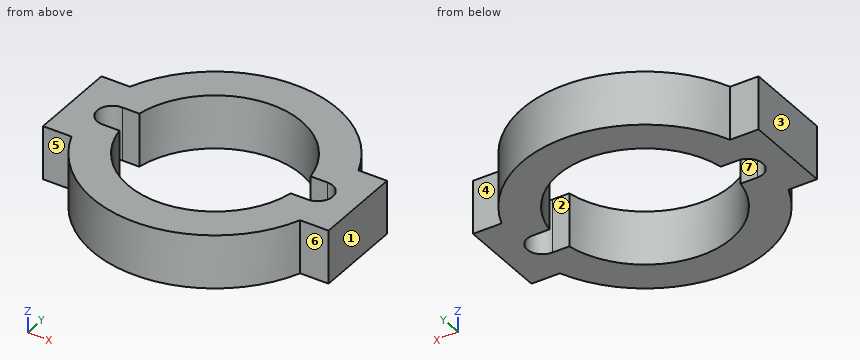
Solid Edge part; units mm, degrees
sketch "Sketch1" plane through (0, 0, 0) normal (0, 0, 1) x (1, 0, 0)
  circle A0 centre (0, 0) radius 13.75
  circle A1 centre (0, 0) radius 9.75
extrude "Protrusion1" add sketch "Sketch1" along normal mid plane 6
sketch "Sketch2" plane through (0, 0, 0) normal (0, 0, 1) x (1, 0, 0)
  line L0 (-11.5, 0) -> (-11.5, 5)
  line L1 (-11.5, 5) -> (-16, 5)
  line L2 (-16, 5) -> (-16, -5)
  line L3 (-16, -5) -> (-11.5, -5)
  line L4 (-11.5, -5) -> (-11.5, 0)
extrude "ExtrudedProtrusion_2" add sketch "Sketch2" along normal mid plane 6
sketch "Sketch3" plane through (-1.125, 0, 3) normal (0, 0, 1) x (0, -1, 0)
  line L0 (-1.7, -10.375) -> (-1.7, -6.9571)
  line L1 (-1.7, -6.9571) -> (1.7, -6.9571)
  line L2 (1.7, -6.9571) -> (1.7, -10.375)
  arc A0 (1.7, -10.375) -> (-1.7, -10.375) centre (0, -10.375) cw
extrude "Cutout1" cut sketch "Sketch3" along normal through all and the other way through all
mirror "Mirror1" about plane through (0, 0, 0) normal (1, 0, 0) of "ExtrudedProtrusion_2", "Cutout1"
CAD build for the part. Positions are in the model's coordinates, mm. Face numbers are marked on the shaded views. A direction names the side the tool comes from. Give positions to 0.01 mm unless a question says otherwise; leave off trailing zeros. Order: outer loops, then holes, each group sorted by start corner. A loop starts at its lowest first (then second) coordinate and runs counter-clockwise, first axis right, second up. Notation, with made-up numbers: (-22.75, 22.25) - (23.25, 22.25) arc R36 ccw to (23.25, 56.25) - close; hole circle Ø10 at (84.5, 46). An arc over 180 degrees is marked (long way). Write each question's results on one line, items separated by ' | '.
1. Pin check, flat tips, straight feed: pin 1 (3.5 mm diameter, centred on x = 15, z = 0, fed in from -Y); pin 2 (1.5 mm diameter, centred on x = 9.5, z = -0.5, fed in from -Y); pin 3 (12 mm diameter, centred on x = 3.5, y = -9, fed in from -Z); pin 4 (1 mm diameter, centred on x = 14.5, z = -1, fed in from +Y). Stop position of each tip, or through.
Calculated:
pin 1: stops at y = -5 | pin 2: stops at y = -10.61 | pin 3: stops at z = -3 | pin 4: stops at y = 5
2. Saw through at C-C on z = -0.65. List the corners of the cut face in (x, y).
Calculated:
outline: (-16, -5) - (-12.81, -5) arc R13.75 ccw to (12.81, -5) - (16, -5) - (16, 5) - (12.81, 5) arc R13.75 ccw to (-12.81, 5) - (-16, 5) - close; hole (-11.5, -1.7) - (-9.6, -1.7) arc R9.75 ccw to (9.6, -1.7) - (11.5, -1.7) arc R1.7 ccw to (11.5, 1.7) - (9.6, 1.7) arc R9.75 ccw to (-9.6, 1.7) - (-11.5, 1.7) arc R1.7 ccw to start
3. Saw through at B-B on x = 5. List the corners of the cut face in (y, z).
Calculated:
outline: (-12.81, -3) - (-8.37, -3) - (-8.37, 3) - (-12.81, 3) - close; (8.37, -3) - (12.81, -3) - (12.81, 3) - (8.37, 3) - close
4. Saw through at A-A on y = 0. List the corners of the cut face in (x, z).
Calculated:
outline: (-16, -3) - (-13.2, -3) - (-13.2, 3) - (-16, 3) - close; (13.2, -3) - (16, -3) - (16, 3) - (13.2, 3) - close
5. Saw through at D-D on y = 10.5. List the corners of the cut face in (x, z).
Calculated:
outline: (-8.88, -3) - (8.88, -3) - (8.88, 3) - (-8.88, 3) - close
6. Probe L1, parallel to X at y = 4, z = -0.55; L2, parallel to X at y = -3.5, z = 1; L3, parallel to Y at x = 6, z = 0.95. List the from-to ranges inside material, lowest first. Write a range as from..to.
Calculated:
L1: x = -16..-8.89, 8.89..16 | L2: x = -16..-9.1, 9.1..16 | L3: y = -12.37..-7.69, 7.69..12.37
7. Pull direction X, two halves, no side cores. Call the marked faces 1, 2, 3 and 4: released by +X, released by -X, zero draft, split by the parting line, or undercut.
Calculated:
face 1: released by +X | face 2: undercut | face 3: released by -X | face 4: zero draft
8. 3-axis set-ups, long thin cutter, end or side, ignore diameter. For the marked faces 5, 6 and 7: which of +Z, -Z, +X, -X, +Y, -Y reach the whole face in a straight line?
Calculated:
face 5: +Z, -Z, -X, -Y | face 6: +Z, -Z, +X, -Y | face 7: +Z, -Z
